Part model, mm, in its own coordinate system. Face numbers are marked on the shaded views. A direction names the side the tool comes from. Round coordinates to 2 decimals unless told otherwise and drop trailing zeros. Write each loop counter-clockwise with the first axis right and the second up, starting at its lowest first coordinate (ties: lowest second). Pieces come first, ordered by that corner, then holes. Notation, with made-up numbers: M 3.5,48 L 54.5,48 A13 cw 54.5,72 Z; hole C 40.25,-4 d11. An arc over 180 degrees is marked long. Use a Markdown table: item, result. Add a question column.
1) Wall check: probe 1 along Y at (x, z) = (-3, 9.75); probe 2 along X at (y, z) = (-14, 7.25); probe 3 along X at (y, z) = (24, 9.25). Give the ranges that are in metal, low to high.
2) Slice it at A-A on x = -10. Write the cut outline in (y, z).
3) Slice it at C-C on z = 11.25. Write the cut outline in (x, y), plus the area to 3 significant figures.
4) Which spindle directions (+Z, -Z, +X, -X, +Y, -Y) get a long thin tool onto all of the face, cutting with end or side? Do the marked faces 4, 5, 6, 7 and 8. Say none if no direction does.
5) Two-plate mould, pull along Y, no slides. Class the marked faces 1, 2 and 3: released by +Y, released by -Y, zero draft, split by the parting line, or undercut.
6) Slice it at B-B on y = -9. Write the cut outline in (x, z), plus the area to 3 significant figures.
7) Drop flat-ended pins along their axis: P1, Ø5, axis at y = 16, z = 4.5, coming from the -X side; P2, Ø11, axis at y = -1.5, z = 5.5, coming from the +X side; P3, Ø0.8, axis at y = -18.5, z = 15, coming from the -X side; P4, Ø2, axis at y = -1, z = 11.5, coming from the -X side. Give the stop position or say it passes through.
```python
from build123d import *

# Parameters (mm, degrees)
F0_W     = 2
F0_H     = 4
F0_H_2   = 2.8740456328
F1_DEPTH = 10
F2_R     = 0.99999
F0_W_2   = 26
F0_H_3   = 7
F3_DEPTH = 2
F4_W     = 24.9721305105
F4_H     = 10
F5_DEPTH = 1.5


# Not quite as in the source:
# - a fillet or chamfer is up to 0.001 mm smaller than in the source, because OpenCascade refuses the exact size


with BuildPart() as f1:
    # F0 (on Top) → F1 (new body)
    with BuildSketch(Plane.XY):
        Polygon((14.5, 18.75), (-14.5, 18.75), (-14.5, 13.8759543672), (-14.5, 9.8759543672), (-14.5, -18.75), (14.5, -18.75), (14.5, 9.8759543672), (14.5, 13.8759543672), align=None)
        Polygon((-13, 4.7144976147), (-13, 17.25), (13, 17.25), (13, 4.7144976147), (13, -2.2855023853), (13, -17.25), (-13, -17.25), (-13, -2.2855023853), align=None, mode=Mode.SUBTRACT)
        with Locations((-15.5, 11.8759543672)):
            Rectangle(F0_W, F0_H)
        Polygon((-16.5, 9.8759543672), (-16.5, 13.8759543672), (-16.5, 29.8609879265), (-19.8, 24.85), (-18, 24.85), (-18, 12.75), (-18, 9.8759543672), align=None)
        with Locations((15.5, 11.8759543672)):
            Rectangle(F0_W, F0_H)
        Polygon((16.5, 29.8609879265), (16.5, 13.8759543672), (16.5, 9.8759543672), (18, 9.8759543672), (18, 12.75), (18, 24.85), (19.8, 24.85), align=None)
        with Locations((-19, 11.3129771836)):
            Rectangle(F0_W, F0_H_2)
        with Locations((19, 11.3129771836)):
            Rectangle(F0_W, F0_H_2)
    extrude(amount=F1_DEPTH)

    # F2 (radius 1 in the source; OpenCascade refuses exactly that, so slightly less here)
    f2_edges = [f1.edges().sort_by_distance(p)[0] for p in [
        (-14.5, 18.75, 5),
        (-20, 9.875954, 5),
        (14.5, 18.75, 5),
        (20, 9.875954, 5),
        (-13, 17.25, 5),
        (14.5, 9.875954, 5),
        (14.5, -18.75, 5),
        (-14.5, -18.75, 5),
        (-13, -17.25, 5),
        (13, 17.25, 5),
        (13, -17.25, 5),
        (-14.5, 13.875954, 5),
        (16.5, 13.875954, 5),
        (-16.5, 13.875954, 5),
        (14.5, 13.875954, 5),
        (-16.5, 29.860988, 5),
        (16.5, 29.860988, 5),
    ]]
    fillet(f2_edges, radius=F2_R)

    # F0 (on Top) → F3 (join)
    with BuildSketch(Plane.XY):
        with Locations((0, 1.2144976147)):
            Rectangle(F0_W_2, F0_H_3)
    extrude(amount=F3_DEPTH)

    # F4 (on face) → F5 (join)
    with BuildSketch(Plane.XZ.offset(18.75)):
        with Locations((0, 15)):
            Rectangle(F4_W, F4_H)
    extrude(amount=-F5_DEPTH)


solid = f1.part
```
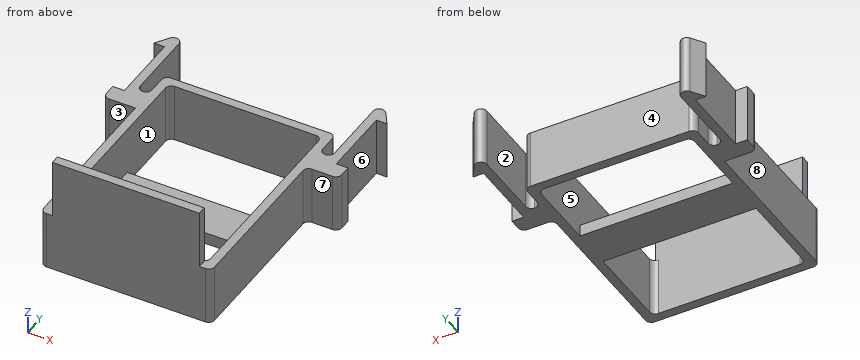
Entries:
| question | item | result |
|---|---|---|
| 1 | probe 1 | y = -18.75 to -17.25, 17.25 to 18.75 |
| 1 | probe 2 | x = -14.5 to -13, 13 to 14.5 |
| 1 | probe 3 | x = -18 to -16.5, 16.5 to 18 |
| 2 | outline | M -18.75,0 L -17.25,0 L -17.25,20 L -18.75,20 Z; M -2.29,0 L 4.71,0 L 4.71,2 L -2.29,2 Z; M 17.25,0 L 18.75,0 L 18.75,10 L 17.25,10 Z |
| 3 | outline | M -12.49,-18.75 L 12.49,-18.75 L 12.49,-17.25 L -12.49,-17.25 Z |
| 3 | area | 37.5 mm^2 |
| 4 | face 4 | +Z, -Z, +Y |
| 4 | face 5 | +Z |
| 4 | face 6 | +Z, -Z, +X |
| 4 | face 7 | +Z, -Z, +X, -Y |
| 4 | face 8 | +Z, -Z, -X, -Y |
| 5 | face 1 | undercut |
| 5 | face 2 | zero draft |
| 5 | face 3 | released by -Y |
| 6 | outline | M -14.5,0 L -13,0 L -13,10 L -14.5,10 Z; M 13,0 L 14.5,0 L 14.5,10 L 13,10 Z |
| 6 | area | 30.0 mm^2 |
| 7 | P1 | stops at x = -18 |
| 7 | P2 | stops at x = 14.5 |
| 7 | P3 | stops at x = -12.49 |
| 7 | P4 | passes through |
